Input: part model. Units: mm. Frame: model coordinates. Face numbers are marked on the shaded views. A direction names the side the tool comes from. Round coordinates to 2 decimals unless told otherwise and drop trailing zeros. Loops run counter-clockwise (first coordinate to the right, second up) from the corner with the lowest first, then second, coordinate; pieces in that order, holes last. Notation, with made-up numbers: M 66.5,-19 L 100.5,-19 A20 cw 100.5,1 Z; hole C 22,-20.75 d8. An arc over 180 degrees is marked long. Use one line per item in the form item = value. Start each with the question number.
Q1. Section query B-B, the plane y = 2.7. Output: boundary loops of the cut face in (x, z).
Q2. Ray query, line 1 along X through (y, z) = (3.55, 0); line 2 along Z through (x, y) = (-27.5, 2.4); line 3 along Z through (x, y) = (23, 0.6). Return the intervals inside material, ascending.
Q3. Access query for the marked faces 5, 6, 7 and 8. Directions: +Z, -Z, +X, -X, +Y, -Y. A direction counts if a zero-diameter tool reaches every point of the face in a straight line with its end or side. Return the directions, or none.
Q4. Section query A-A, the plane x = 0. Output: boundary loops of the cut face in (y, z), and give its area (3 significant figures).
Q5. Section query C-C, the plane z = 0. Output: boundary loops of the cut face in (x, y), and give its area (3 significant figures).
Q6. Section query D-D, the plane x = 25.5. Output: boundary loops of the cut face in (y, z), and give its area (3 significant figures).
Q7. Mould query, pull axis X, two halves, no side actions, for the marked faces 1, 2, 3 and 4. Classes: pulls with the +X half, pulls with the -X half, needs draft (parallel to the pull), parting line crosses it, or undercut.
Q8. First-contact query: P1, Ø1.6, axis at x = -27.5, z = 0, coming from the +Y side; P2, Ø1, axis at x = 11, y = 3.5, coming from the -Z side; P3, Ø2, axis at x = 18, y = 2, coming from the +Z side; P4, Ø1, axis at y = 2.5, z = -2, coming from the +X side. Flat tips, straight axial feed; report the tip coordinate or a pass-through.
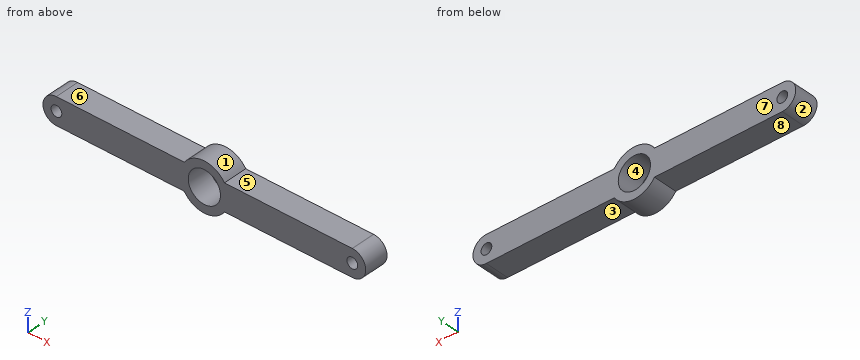
```python
from build123d import *

# Parameters (mm, degrees)
BOSS_EXTRUDE2_DEPTH     = 4.5
SKETCH2_R               = 3
CUT_EXTRUDE1_DEPTH      = 5.5
CUT_EXTRUDE1_DEPTH_BACK = 1
SKETCH3_R               = 1
CUT_EXTRUDE2_DEPTH      = 5.5
CUT_EXTRUDE2_DEPTH_BACK = 1


with BuildPart() as part:
    # Sketch1 → Boss-Extrude2 (new body)
    with BuildSketch(Plane(origin=(0, 0, 0), x_dir=(1, 0, 0), z_dir=(0, 1, 0))):
        with BuildLine():
            Line((-3.741657387, 2.5), (-27.5, 2.5))
            ThreePointArc((-27.5, 2.5), (-30, 0), (-27.5, -2.5))
            Line((-27.5, -2.5), (-3.741657387, -2.5))
            ThreePointArc((-3.741657387, -2.5), (0, -4.5), (3.741657387, -2.5))
            Line((3.741657387, -2.5), (27.5, -2.5))
            ThreePointArc((27.5, -2.5), (30, 0), (27.5, 2.5))
            Line((27.5, 2.5), (3.741657387, 2.5))
            ThreePointArc((3.741657387, 2.5), (0, 4.5), (-3.741657387, 2.5))
        make_face()
    extrude(amount=BOSS_EXTRUDE2_DEPTH)

    # Sketch2 → Cut-Extrude1 (cut, two sides)
    with BuildSketch(Plane(origin=(0, 0, 0), x_dir=(1, 0, 0), z_dir=(0, 1, 0))) as cut_extrude1_sk:
        Circle(SKETCH2_R)
    extrude(amount=CUT_EXTRUDE1_DEPTH, mode=Mode.SUBTRACT)
    extrude(cut_extrude1_sk.sketch, amount=-CUT_EXTRUDE1_DEPTH_BACK, mode=Mode.SUBTRACT)

    # Sketch3 → Cut-Extrude2 (cut, two sides)
    with BuildSketch(Plane(origin=(0, 0, 0), x_dir=(1, 0, 0), z_dir=(0, 1, 0))) as cut_extrude2_sk:
        with Locations((-27.5, 0)):
            Circle(SKETCH3_R)
        with Locations((27.5, 0)):
            Circle(SKETCH3_R)
    extrude(amount=CUT_EXTRUDE2_DEPTH, mode=Mode.SUBTRACT)
    extrude(cut_extrude2_sk.sketch, amount=-CUT_EXTRUDE2_DEPTH_BACK, mode=Mode.SUBTRACT)


solid = part.part
```
Results found:
q1.outline = M -27.5,-2.5 L -3.74,-2.5 A4.5 ccw 3.74,-2.5 L 27.5,-2.5 A2.5 ccw 27.5,2.5 L 3.74,2.5 A4.5 ccw -3.74,2.5 L -27.5,2.5 A2.5 ccw Z; hole C -27.5,0 d2; hole C 0,0 d6; hole C 27.5,0 d2
q2.line_1 = -30 to -28.5, -26.5 to -3, 3 to 26.5, 28.5 to 30
q2.line_2 = -2.5 to -1, 1 to 2.5
q2.line_3 = -2.5 to 2.5
q3.face_5 = +Z, +X, +Y, -Y
q3.face_6 = +Z, -X, +Y, -Y
q3.face_7 = +Z, -Z, +X, -X, +Y
q3.face_8 = -Z, -X, +Y, -Y
q4.outline = M 0,-4.5 L 4.5,-4.5 L 4.5,-3 L 0,-3 Z; M 0,3 L 4.5,3 L 4.5,4.5 L 0,4.5 Z
q4.area = 13.5 mm²
q5.outline = M -30,0 L -28.5,0 L -28.5,4.5 L -30,4.5 Z; M -26.5,0 L -3,0 L -3,4.5 L -26.5,4.5 Z; M 3,0 L 26.5,0 L 26.5,4.5 L 3,4.5 Z; M 28.5,0 L 30,0 L 30,4.5 L 28.5,4.5 Z
q5.area = 225 mm²
q6.outline = M 0,-2.5 L 4.5,-2.5 L 4.5,2.5 L 0,2.5 Z
q6.area = 22.5 mm²
q7.face_1 = parting line crosses it
q7.face_2 = pulls with the -X half
q7.face_3 = needs draft
q7.face_4 = undercut
q8.P1 = through
q8.P2 = -2.5
q8.P3 = 2.5
q8.P4 = 29.5
